from build123d import *

# Parameters (mm, degrees)
SKETCH1_W      = 171.45
SKETCH1_H      = 1.905
EXTRUDE1_DEPTH = 88.9
SKETCH2_W      = 155.575
SKETCH2_H      = 133.35
EXTRUDE2_DEPTH = 22.1
FILLET1_R      = 10
FILLET2_R      = 10


with BuildPart() as part:
    # Sketch1 → Extrude1 (new body, symmetric)
    with BuildSketch(Plane.XY):
        with Locations((0, 0.9525)):
            Rectangle(SKETCH1_W, SKETCH1_H)
    extrude(amount=EXTRUDE1_DEPTH, both=True)

    # Sketch2 → Extrude2 (add)
    with BuildSketch(Plane.XZ):
        with Locations((0, -15.875)):
            Rectangle(SKETCH2_W, SKETCH2_H)
    extrude(amount=EXTRUDE2_DEPTH)

    # Fillet1
    fillet1_edges = [part.edges().sort_by_distance(p)[0] for p in [
        (-77.7875, -11.05, 50.8),
        (-77.7875, -11.05, -82.55),
        (77.7875, -11.05, -82.55),
        (77.7875, -11.05, 50.8),
    ]]
    fillet(fillet1_edges, radius=FILLET1_R)

    # Fillet2
    fillet2_edges = [part.edges().sort_by_distance(p)[0] for p in [
        (0, -22.1, -82.55),
        (-77.7875, -22.1, -15.875),
        (77.7875, -22.1, -15.875),
        (0, -22.1, 50.8),
        (-74.858567812, -22.1, 47.871067812),
        (74.858567812, -22.1, 47.871067812),
        (74.858567812, -22.1, -79.621067812),
        (-74.858567812, -22.1, -79.621067812),
    ]]
    fillet(fillet2_edges, radius=FILLET2_R)


solid = part.part
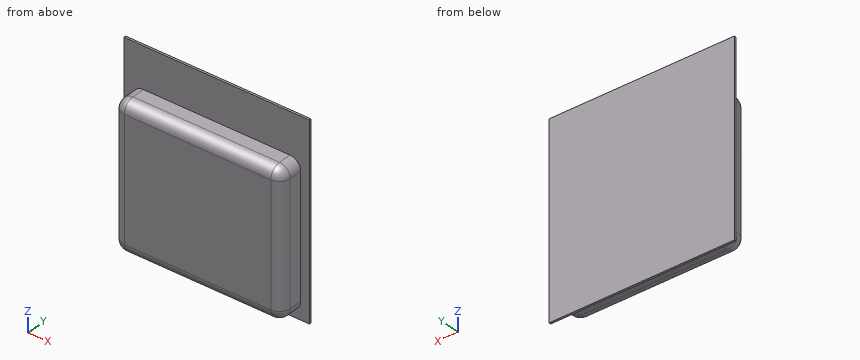
Geometry check sheet. Reference: the model listing, model coordinates, mm. Give positions to 0.01 mm unless a question says otherwise; leave off trailing zeros. Write each loop counter-clockwise with the first axis right and the second up, starting at its lowest first coordinate (ties: lowest second). Pieces come first, ordered by that corner, then holes.
1) Thickness scan on line 1 (Z direction, x = 0.5, y = -13); line 2 (X direction, y = -0.25, z = 41); line 3 (Z direction, x = -39.5, y = -10.25). Record the ranges inside material, lowest first.
Values follow:
line 1: z = -82.51 to 50.76
line 2: x = -77.79 to 77.79
line 3: z = -82.55 to 50.8
2) Cross-section at B-B (z = -5). Record the boundary of the cut face in (x, y) (1 decimal).
Values follow:
outline: (-85.7, 0) - (-77.8, 0) - (-77.8, -12.1) arc R10 ccw to (-67.8, -22.1) - (67.8, -22.1) arc R10 ccw to (77.8, -12.1) - (77.8, 0) - (85.7, 0) - (85.7, 1.9) - (-85.7, 1.9) - close
3) Cross-section at D-D (y = -15.5). Record the boundary of the cut face in (x, z), plus the area to 3 significant figures.
Values follow:
outline: (-77.19, -72.55) arc R9.4 ccw to (-67.79, -81.95) - (67.79, -81.95) arc R9.4 ccw to (77.19, -72.55) - (77.19, 40.8) arc R9.4 ccw to (67.79, 50.2) - (-67.79, 50.2) arc R9.4 ccw to (-77.19, 40.8) - close
area: 20,300 mm2
4) Cross-section at A-A (y = -5.5). Record the boundary of the cut face in (x, z), plus the area to 3 significant figures.
Values follow:
outline: (-77.79, -72.55) arc R10 ccw to (-67.79, -82.55) - (67.79, -82.55) arc R10 ccw to (77.79, -72.55) - (77.79, 40.8) arc R10 ccw to (67.79, 50.8) - (-67.79, 50.8) arc R10 ccw to (-77.79, 40.8) - close
area: 20,700 mm2
5) Go/stop test with flat-tipped pins: pin 1 Ø3.5 at (y, z) = (-8, 4) entering from +X; pin 2 Ø1.5 at (y, z) = (-6.5, 37) entering from -X; pin 3 Ø2 at (x, y) = (48, -10.5) entering from -Z. Record where each tip stops, or that it passes through.
Values follow:
pin 1: stops at x = 77.79
pin 2: stops at x = -77.79
pin 3: stops at z = -82.55
6) Cross-section at C-C (x = -62.5). Record the boundary of the cut face in (y, z) (3 decimals), plus the area to 3 significant figures.
Values follow:
outline: (-22.1, -72.55) arc R10 ccw to (-12.1, -82.55) - (0, -82.55) - (0, -88.9) - (1.905, -88.9) - (1.905, 88.9) - (0, 88.9) - (0, 50.8) - (-12.1, 50.8) arc R10 ccw to (-22.1, 40.8) - close
area: 3,240 mm2
